Build history of the part. All positions in model axes, mm. Face numbers are marked on the shaded views. A direction names the side the tool comes from. Give positions to 0.01 mm unless a question says otherwise; leave off trailing zeros. Write each loop counter-clockwise with the first axis right and the second up, starting at its lowest first coordinate (ties: lowest second). Pieces come first, ordered by that corner, then holes. Notation, with made-up numbers: (78.5, 59.25) -> (112.5, 59.25) arc R20 ccw to (112.5, 76.25) -> close; hole circle Ø5 at (83.5, 16.25). An arc over 180 degrees is marked (long way). Write item = value, one per line. Start each with the question number.
Q1. Tool access for the marked faces 5 and 6: list every direction of +Z, -Z, +X, -X, +Y, -Y with a clear straight run to the whole face (end or side of a thin tool).
Q2. Saw through at B-B, the plane y = -16. List the corners of the cut face in (x, z), then the cut area to 3 significant figures.
Q3. Saw through at D-D, the plane x = -14. Give the number of separate pieces and of enclosed holes in the cut face, then the cut area to 3 significant figures.
Q4. Saw through at A-A, the plane z = -34. List the corners of the cut face in (x, y), then the cut area to 3 significant figures.
Q5. Drop flat-ended pins along their axis: P1, Ø7, axis at x = -9, y = 0, coming from the +Z side; P2, Ø5, axis at x = 19, z = -57.5, coming from the +Y side; P3, Ø8, axis at x = 9, z = -14.5, coming from the -Y side; P4, Ø12, axis at y = -5.5, z = -43, coming from the +X side. Give the stop position or say it passes through.
Q6. Wall check: line 1 (Y direction, x = 18, z = 2.9); line 2 (X direction, y = 2.5, z = -21); line 3 (X direction, y = 16, z = -72). Give the ranges that are in metal, low to high.
Q7. Saw through at C-C, the plane z = -11. List the corners of the cut face in (x, y).
Q8. Mould opens along Y. For the marked faces 1, 2, 3 and 4 say: pulls with the +Y half, pulls with the -Y half, needs draft (parallel to the pull), parting line crosses it, or undercut.
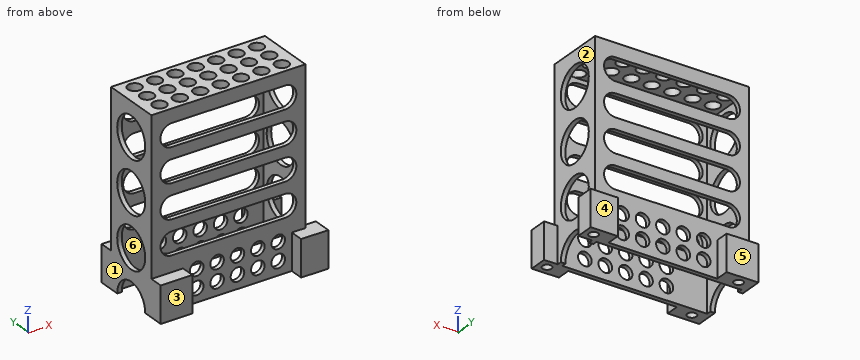
from build123d import *

# Parameters (mm, degrees)
SKICA1_W                 = 68
SKICA1_H                 = 26
P_IDAT_VYSUNUT_M1_DEPTH  = 4
SKICA2_W                 = 68
SKICA2_H                 = 26
SKICA2_W_2               = 64
SKICA2_H_2               = 22
P_IDAT_VYSUNUT_M2_DEPTH  = 80
P_IDAT_VYSUNUT_M9_DEPTH  = 16
SKICA3_R                 = 2
ODEBRAT_VYSUNUT_M1_DEPTH = 15
ODEBRAT_VYSUNUT_M2_DEPTH = 95.994736696
SKICA5_R                 = 9
ODEBRAT_VYSUNUT_M3_DEPTH = 111.620974503
SKICA8_W                 = 48
SKICA8_H                 = 6
ODEBRAT_VYSUNUT_M4_DEPTH = 16
SKICA9_R                 = 3
ODEBRAT_VYSUNUT_M5_DEPTH = 4
SKICA10_R                = 3
ODEBRAT_VYSUNUT_M6_DEPTH = 95.994736696


with BuildPart() as part:
    # Skica1 → Přidat vysunutím1 (new body)
    with BuildSketch(Plane.XY):
        Rectangle(SKICA1_W, SKICA1_H)
    extrude(amount=P_IDAT_VYSUNUT_M1_DEPTH)

    # Skica2 → Přidat vysunutím2 (add)
    with BuildSketch(Plane(origin=(0, 0, 0), x_dir=(-1, 0, 0), z_dir=(0, 0, -1))):
        Rectangle(SKICA2_W, SKICA2_H)
        Rectangle(SKICA2_W_2, SKICA2_H_2, mode=Mode.SUBTRACT)
    extrude(amount=P_IDAT_VYSUNUT_M2_DEPTH)

    # Skica7 → Přidat vysunutím9 (add)
    with BuildSketch(Plane.XY.offset(-80)):
        Polygon((3, 19), (40, 19), (40, 11), (34, 11), (34, 13), (-34, 13), (-34, 19), align=None)
        Polygon((-34, -19), (-34, -13), (34, -13), (34, -11), (40, -11), (40, -19), (3, -19), align=None)
    extrude(amount=P_IDAT_VYSUNUT_M9_DEPTH)

    # Skica3 → Odebrat vysunutím1 (cut)
    with BuildSketch(Plane(origin=(0, 0, -80), x_dir=(-1, 0, 0), z_dir=(0, 0, -1))):
        with Locations((-36, 15)):
            Circle(SKICA3_R)
        with Locations(Location((28, 15, 0), (0, 0, 180))):
            Circle(SKICA3_R)
        with Locations((28, -15)):
            Circle(SKICA3_R)
        with Locations(Location((-36, -15, 0), (0, 0, 180))):
            Circle(SKICA3_R)
    extrude(amount=-ODEBRAT_VYSUNUT_M1_DEPTH, mode=Mode.SUBTRACT)

    # Skica4 → Odebrat vysunutím2 (cut, through all)
    with BuildSketch(Plane.XZ.offset(13)):
        with BuildLine():
            Line((-25, -57), (25, -57))
            ThreePointArc((25, -57), (30, -52), (25, -47))
            Line((25, -47), (-25, -47))
            ThreePointArc((-25, -47), (-30, -52), (-25, -57))
        make_face()
        with BuildLine():
            Line((-25, -32), (25, -32))
            ThreePointArc((25, -32), (30, -37), (25, -42))
            Line((25, -42), (-25, -42))
            ThreePointArc((-25, -42), (-30, -37), (-25, -32))
        make_face()
        with BuildLine():
            Line((-25, -17), (25, -17))
            ThreePointArc((25, -17), (30, -22), (25, -27))
            Line((25, -27), (-25, -27))
            ThreePointArc((-25, -27), (-30, -22), (-25, -17))
        make_face()
        with BuildLine():
            Line((-25, -2), (25, -2))
            ThreePointArc((25, -2), (30, -7), (25, -12))
            Line((25, -12), (-25, -12))
            ThreePointArc((-25, -12), (-30, -7), (-25, -2))
        make_face()
    extrude(amount=-ODEBRAT_VYSUNUT_M2_DEPTH, mode=Mode.SUBTRACT)

    # Skica5 → Odebrat vysunutím3 (cut, through all)
    with BuildSketch(Plane.ZY.offset(34)):
        with Locations((-80, 0)):
            Circle(SKICA5_R)
        with Locations((-57, 0)):
            Circle(SKICA5_R)
        with Locations((-34, 0)):
            Circle(SKICA5_R)
        with Locations((-11, 0)):
            Circle(SKICA5_R)
    extrude(amount=-ODEBRAT_VYSUNUT_M3_DEPTH, mode=Mode.SUBTRACT)

    # Skica8 → Odebrat vysunutím4 (cut)
    with BuildSketch(Plane(origin=(0, 0, -80), x_dir=(-1, 0, 0), z_dir=(0, 0, -1))):
        with Locations((-4, 16)):
            Rectangle(SKICA8_W, SKICA8_H)
        with Locations((-4, -16)):
            Rectangle(SKICA8_W, SKICA8_H)
    extrude(amount=-ODEBRAT_VYSUNUT_M4_DEPTH, mode=Mode.SUBTRACT)

    # Skica9 → Odebrat vysunutím5 (cut)
    with BuildSketch(Plane.XY.offset(4)):
        with Locations((-27, 8)):
            Circle(SKICA9_R)
        with Locations((-18, 8)):
            Circle(SKICA9_R)
        with Locations((-9, 8)):
            Circle(SKICA9_R)
        with Locations((0, 8)):
            Circle(SKICA9_R)
        with Locations((9, 8)):
            Circle(SKICA9_R)
        with Locations((18, 8)):
            Circle(SKICA9_R)
        with Locations((27, 8)):
            Circle(SKICA9_R)
        with Locations((-18, 0)):
            Circle(SKICA9_R)
        with Locations((-9, 0)):
            Circle(SKICA9_R)
        Circle(SKICA9_R)
        with Locations((9, 0)):
            Circle(SKICA9_R)
        with Locations((18, 0)):
            Circle(SKICA9_R)
        with Locations((27, 0)):
            Circle(SKICA9_R)
        with Locations((-18, -8)):
            Circle(SKICA9_R)
        with Locations((-9, -8)):
            Circle(SKICA9_R)
        with Locations((0, -8)):
            Circle(SKICA9_R)
        with Locations((9, -8)):
            Circle(SKICA9_R)
        with Locations((18, -8)):
            Circle(SKICA9_R)
        with Locations((27, -8)):
            Circle(SKICA9_R)
        with Locations((-27, 0)):
            Circle(SKICA9_R)
        with Locations((-27, -8)):
            Circle(SKICA9_R)
    extrude(amount=-ODEBRAT_VYSUNUT_M5_DEPTH, mode=Mode.SUBTRACT)

    # Skica10 → Odebrat vysunutím6 (cut, through all)
    with BuildSketch(Plane(origin=(0, 13, 0), x_dir=(1, 0, 0), z_dir=(0, 1, 0))):
        with Locations(Location((-14, 74, 0), (0, 0, 270))):
            Circle(SKICA10_R)
        with Locations(Location((-5, 74, 0), (0, 0, 270))):
            Circle(SKICA10_R)
        with Locations(Location((4, 74, 0), (0, 0, 270))):
            Circle(SKICA10_R)
        with Locations(Location((13, 74, 0), (0, 0, 270))):
            Circle(SKICA10_R)
        with Locations(Location((22, 74, 0), (0, 0, 270))):
            Circle(SKICA10_R)
        with Locations(Location((-5, 66, 0), (0, 0, 270))):
            Circle(SKICA10_R)
        with Locations(Location((4, 66, 0), (0, 0, 270))):
            Circle(SKICA10_R)
        with Locations(Location((13, 66, 0), (0, 0, 270))):
            Circle(SKICA10_R)
        with Locations(Location((22, 66, 0), (0, 0, 270))):
            Circle(SKICA10_R)
        with Locations(Location((-14, 66, 0), (0, 0, 270))):
            Circle(SKICA10_R)
    extrude(amount=-ODEBRAT_VYSUNUT_M6_DEPTH, mode=Mode.SUBTRACT)


solid = part.part
Report:
q1.face_5 = +Z, -Z, +X, -X, +Y
q1.face_6 = -Z
q2.outline = (-34, -80) -> (-29.73, -80) -> (-29.73, -65) -> (-26.27, -65) -> (-26.27, -80) -> (-20, -80) -> (-20, -64) -> (-34, -64) -> close; (28, -80) -> (34.27, -80) -> (34.27, -65) -> (37.73, -65) -> (37.73, -80) -> (40, -80) -> (40, -64) -> (28, -64) -> close
q2.area = 312 mm2
q3.separate_pieces = 13
q3.enclosed_holes = 0
q3.area = 216 mm2
q4.outline = (-34, -13) -> (-29, -13) -> (-29, -11) -> (-32, -11) -> (-32, -9) -> (-34, -9) -> close; (-34, 9) -> (-32, 9) -> (-32, 11) -> (-29, 11) -> (-29, 13) -> (-34, 13) -> close; (29, -13) -> (34, -13) -> (34, -9) -> (32, -9) -> (32, -11) -> (29, -11) -> close; (29, 11) -> (32, 11) -> (32, 9) -> (34, 9) -> (34, 13) -> (29, 13) -> close
q4.area = 56.0 mm2
q5.P1 = 4
q5.P2 = 13
q5.P3 = -13
q5.P4 = 34
q6.line_1 = -13 to -11, -5 to -3, 3 to 5, 11 to 13
q6.line_2 = -34 to -32, 32 to 34
q6.line_3 = -34 to -29.73, -26.27 to -20, 28 to 34.27, 37.73 to 40
q7.outline = (-34, -13) -> (-28, -13) -> (-28, -11) -> (-32, -11) -> (-32, -9) -> (-34, -9) -> close; (-34, 9) -> (-32, 9) -> (-32, 11) -> (-28, 11) -> (-28, 13) -> (-34, 13) -> close; (28, -13) -> (34, -13) -> (34, -9) -> (32, -9) -> (32, -11) -> (28, -11) -> close; (28, 11) -> (32, 11) -> (32, 9) -> (34, 9) -> (34, 13) -> (28, 13) -> close
q8.face_1 = needs draft
q8.face_2 = undercut
q8.face_3 = pulls with the -Y half
q8.face_4 = pulls with the +Y half
